Check sheet for the modelled part. Datum: model origin and axes. Units: mm. A direction names the side the tool comes from. Give positions to 0.01 mm unless a question says otherwise; leave off trailing zeros. Write each question's results on one line, items separated by ' | '. Start each with the question number.
Item 1: Cross-section at A-A on z = 0. State how many separate pieces and enclosed holes the cut face has, then the cut area to 3 significant figures.
Item 2: Gauge pin test, flat ends, axial feed: pin 1 Ø6 at (x, z) = (-31.5, -24.5) entering from -Y; pin 2 Ø8 at (x, z) = (1, -32.5) entering from +Y; pin 3 Ø1 at (x, y) = (-24, 7.5) entering from -Z; pin 4 Ø3 at (x, y) = (28, 3.5) entering from -Z. Record the tip position at first contact, or that the pin passes through.
Item 3: Access from +Z, -Z, +X, -X, +Y, -Y to the whole of each face (thin tool, end or side, straight path). Record for faces 4 (the face through (-36.11, 1.48, 1.34)), 5 (the face through (-32, 3, 2)), 6 (the face through (0, 7, 0)).
Item 4: Mould release check, pull along Z, two halves, no side actions. Record for faces 1 (the face through (-11, 0, 1)), 2 (the face through (-28, 5, -45)), 3 (the face through (38.88, 5.46, -1.08)): pulls with the +Z half, pulls with the -Z half, needs draft (parallel to the pull), parting line crosses it, or undercut.
Item 5: Scan lines: line 1 along Z through (x, y) = (0, 4.5); line 2 along Z through (x, y) = (0, 1.7); line 3 along Y through (x, z) = (-36.5, -3). Record each from-to range of solid material in increasing order.
Autodesk Inventor part; units mm, degrees
ref_plane "YZ Plane" through (0, 0, 0) normal (1, 0, 0) x (0, 1, 0)
ref_plane "XZ Plane" through (0, 0, 0) normal (0, 1, 0) x (-1, 0, 0)
ref_plane "XY Plane" through (0, 0, 0) normal (0, 0, 1) x (1, 0, 0)
sketch "スケッチ1" plane through (0, 0, 0) normal (0, 1, 0) x (-1, 0, 0)
  circle A0 centre (0, 0) radius 53
  dimension "d0" = 106
extrude "押し出し1" add sketch "スケッチ1" along normal blind 10
sketch "スケッチ2" plane through (0, 10, 0) normal (0, 1, 0) x (1, 0, 0)
  circle A0 centre (0, 0) radius 50.5
  dimension "d3" = 101
extrude "押し出し2" cut sketch "スケッチ2" against normal blind 2
sketch "スケッチ3" plane through (0, 8, 0) normal (0, 1, 0) x (1, 0, 0)
  point P0 (0, 0)
  point P1 (34, 0)
  point P2 (0, 34)
  point P3 (-34, 0)
  point P4 (0, -34)
  dimension "d6" = 34
  dimension "d9" = 360
hole "穴2" at (-34, 8, 0) at (0, 8, -34) at (34, 8, 0) at (0, 8, 34) direction (0, -1, 0) diameter 5 end through all counterbore diameter 10 counterbore depth 5
fillet "フィレット1" radius 0.5 1 edges at (53, 10, 0)
sketch "スケッチ4" plane through (0, 0, 0) normal (0, -1, 0) x (1, 0, 0)
  circle A0 centre (0, 0) radius 6.75
  dimension "d26" = 13.5
extrude "押し出し3" cut sketch "スケッチ4" against normal blind 7
properties part number "GNSS_mount"
Answer sheet:
1) separate pieces: 3 | enclosed holes: 0 | area: 633 mm²
2) pin 1: stops at y = 0 | pin 2: stops at y = 8 | pin 3: stops at z = -47.51 | pin 4: stops at z = -45.9
3) face 4: +Y, -Y | face 5: +Y | face 6: -Y
4) face 1: needs draft | face 2: parting line crosses it | face 3: undercut
5) line 1: z = -53 to -39, -29 to -6.75, 6.75 to 29, 39 to 53 | line 2: z = -53 to -36.5, -31.5 to -6.75, 6.75 to 31.5, 36.5 to 53 | line 3: y = 0 to 3
